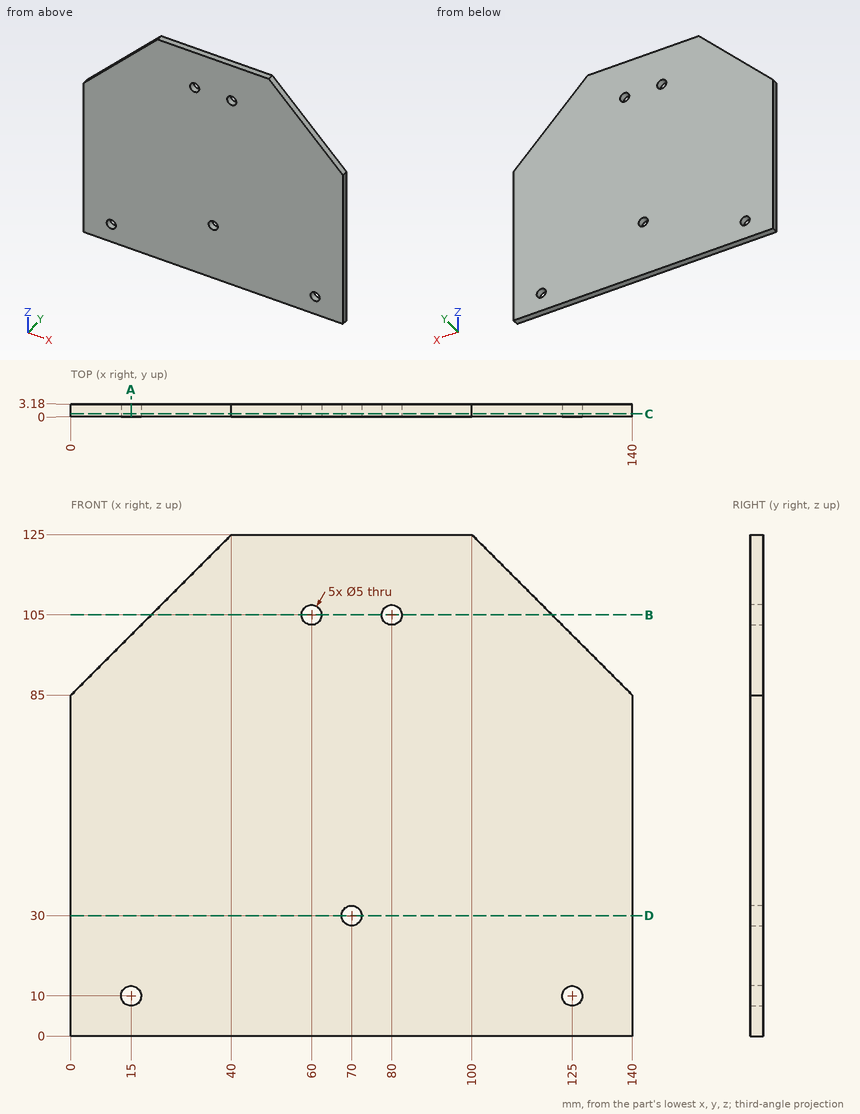
Part print with two shaded views. Sizes in mm from the minimum x, y, z corner. Round coordinates to 2 decimals unless told otherwise and drop trailing zeros. Write each loop counter-clockwise with the first axis right and the second up, starting at its lowest first coordinate (ties: lowest second). Pieces come first, ordered by that corner, then holes. Notation, with made-up numbers: (85.5, 56) -> (120.5, 56) arc R15 cw to (120.5, 68) -> close; hole circle Ø4 at (9.5, 31.25). An arc over 180 degrees is marked (long way). Use one line per item in the form item = value.
Q1. Band-saw the part on C-C, the plane y = 0.7. Write the cut outline in (x, z), then the cut area to 3 significant figures.
Conclusion:
outline = (0, 0) -> (140, 0) -> (140, 85) -> (100, 125) -> (40, 125) -> (0, 85) -> close; hole circle Ø5 at (15, 10); hole circle Ø5 at (60, 105); hole circle Ø5 at (70, 30); hole circle Ø5 at (80, 105); hole circle Ø5 at (125, 10)
area = 15,800 mm²
Q2. Band-saw the part on A-A, the plane x = 15. Write the cut outline in (y, z), then the cut area to 3 significant figures.
Conclusion:
outline = (0, 0) -> (3.18, 0) -> (3.18, 7.5) -> (0, 7.5) -> close; (0, 12.5) -> (3.18, 12.5) -> (3.18, 100) -> (0, 100) -> close
area = 302 mm²
Q3. Band-saw the part on D-D, the plane z = 30. Write the cut outline in (x, y), then the cut area to 3 significant figures.
Conclusion:
outline = (0, 0) -> (67.5, 0) -> (67.5, 3.18) -> (0, 3.18) -> close; (72.5, 0) -> (140, 0) -> (140, 3.18) -> (72.5, 3.18) -> close
area = 429 mm²
Q4. Drill centre lines: L1, parallel to Z at x = 80, y = 1; L2, parallel to Z at x = 125, y = 1.5; L3, parallel to X at y = 1.35, z = 30. Where is each one in solid material? Low to high.
Conclusion:
L1 = 0 to 102.5, 107.5 to 125
L2 = 0 to 7.5, 12.5 to 100
L3 = 0 to 67.5, 72.5 to 140
Q5. Band-saw the part on B-B, the plane z = 105. Write the cut outline in (x, y).
Conclusion:
outline = (20, 0) -> (57.5, 0) -> (57.5, 3.18) -> (20, 3.18) -> close; (62.5, 0) -> (77.5, 0) -> (77.5, 3.18) -> (62.5, 3.18) -> close; (82.5, 0) -> (120, 0) -> (120, 3.18) -> (82.5, 3.18) -> close
